from build123d import *

# Parameters (mm, degrees)
F4_T = -2.5


with BuildPart() as f1:
    # F0 (on Front) → F1 (revolve)
    with BuildSketch(Plane.XZ):
        with BuildLine():
            ThreePointArc((32.4202927587, 23.5130339861), (-9.5793837681, 65.5127105129), (-51.579060295, 23.5130339861))
            Line((-51.579060295, 23.5130339861), (32.4202927587, 23.5130339861))
        make_face()
    revolve(axis=Axis((1.7417054623, 0, 23.5130339861), (1, 0, 0)))

    # F2 (on Front) → F3 (revolve)
    with BuildSketch(Plane.XZ):
        Polygon((-11.5802306682, -112.6956120133), (-11.5802306682, 26.4526642859), (-51.4328964055, 26.4526642859), (-109.681583941, -112.6956120133), align=None)
    revolve(axis=Axis((-11.5802306682, 0, -22.7773860097), (0, 0, -1)))

    # F4
    f4_openings = [f1.faces().sort_by_distance(p)[0] for p in [
        (-11.580231, 0, -112.695612),
    ]]
    offset(amount=F4_T, openings=f4_openings, kind=Kind.INTERSECTION)

    # F6 (on offset) → F7 (join, up to the next surface of F1)
    with BuildSketch(Plane.YZ.offset(100)):
        Polygon((43.8527846002, -20.5623030921), (31.7161967759, -0.4996404972), (11.5647516543, -12.6899358952), (6.7012720683, -40.6980113115), (0.1556711213, -40.6980113115), (-6.3899298257, -40.6980113115), (-11.2534094117, -12.6899358952), (-31.4048545333, -0.4996404972), (-43.5414423575, -20.5623030921), (-29.0120014979, -28.2718026068), (-15.5202871088, -33.4303977157), (-21.773227875, -111.2250647365), (22.0845701176, -111.2250647365), (15.8316293515, -33.4303977157), (29.3233437405, -28.2718026068), align=None)
    extrude(until=Until.NEXT, dir=(-1, 0, 0))


solid = f1.part
Input: part model. Units: mm. Frame: model coordinates. A direction names the side the tool comes from. Give positions to 0.01 mm unless a question says otherwise; leave off trailing zeros. Write each loop counter-clockwise with the first axis right and the second up, starting at its lowest first coordinate (ties: lowest second). Pieces come first, ordered by that corner, then holes. Notation, with made-up numbers: M 28,14.25 L 33,14.25 A12 cw 33,19.25 Z; hole C 41,33 d4. An arc over 180 degrees is marked long. Write item = value, one per line. Start each with the question number.
1) Cut plane B-B on y = 0. Return the cut outline in (x, z), then the cut area to 3 significant figures.
2) Draft query along Y for faces 1 (the flat face through (72.124, 9.167, -26.498)), 2 (the flat face through (72.35, 22.48, -30.89)), 3 (the flat face through (81.46, -17.91, -63.14)). Return one class per face: +Y half, -Y half, draft (parallel to the pull), parting line (faces both ways), or undercut.
3) Cut plane C-C on z = -61. Return the cut outline in (x, y).
4) Reachability of faces 4 (the flat face through (65.01, -36.38, -24.36)), 5 (the flat face through (81.433, 18.307, -64.228)), 6 (the flat face through (64.89, -37.39, -10.39)), 7 (the flat face through (78, 0, -40.698)) from +Z, -Z, +X, -X, +Y, -Y: full face, straight path, thin tool, end or side. Return the list, or none.
5) First-contact query: pin 1 Ø4 at (y, z) = (-33.5, -13.5) entering from -X; pin 2 Ø6 at (x, y) = (24.5, 65.5) entering from +Z; pin 3 Ø5 at (x, y) = (-83, 66.5) entering from +Z. Flat tips, straight axial feed; report the tip coordinate or a pass-through.
6) Material intervals for line 1 along X through (y, z) = (-11.5, 28.5); line 2 along Y through (x, z) = (51.5, -54.5); line 3 along X through (y, z) = (3.5, -86), sorted ascending. Write a range as [from, to].
7) Cut plane A-A on z = -17.5. Return the cut outline in (x, y), then the cut area to 3 significant figures.
8) Cut plane D-D on z = -90. Return the cut outline in (x, y).
Solved:
q1.outline = M -109.68,-112.7 L -106.97,-112.7 L -49.02,25.75 A39.5 cw long 29.42,17.24 L 83.81,-112.7 L 86.52,-112.7 L 85.91,-111.23 L 100,-111.23 L 100,-40.7 L 56.38,-40.7 L 32,17.56 A42 ccw long -51.48,26.33 Z
q1.area = 3,090 mm2
q2.face_1 = undercut
q2.face_2 = +Y half
q2.face_3 = -Y half
q3.outline = M 62.72,18.05 A76.46 ccw long 62.8,-17.74 L 100,-17.74 L 100,18.05 Z; hole C -11.58,0 d147.5
q4.face_4 = +X, -Y
q4.face_5 = +X, +Y
q4.face_6 = +Z, +X, -Y
q4.face_7 = +Z, +X
q5.pin_1 = -58.91
q5.pin_2 = -49.82
q5.pin_3 = -105.49
q6.line_1 = [-49.66, -47.04], [27.88, 30.51]
q6.line_2 = [-38.19, -32.65], [32.65, 38.19]
q6.line_3 = [-98.44, -95.72], [72.56, 100]
q7.outline = M 28.78,42 A58.25 ccw long 29.1,-41.69 L 100,-41.69 L 100,-10.42 L 45.73,-10.42 A58.25 ccw 45.67,10.73 L 100,10.73 L 100,42 Z; hole C -11.58,0 d111.08
q7.area = 4,760 mm2
q8.outline = M 74.65,20.38 A88.6 ccw long 74.72,-20.07 L 100,-20.07 L 100,20.38 Z; hole C -11.58,0 d171.78
